from build123d import *

# Parameters (mm, degrees)
BOSS_EXTRUDE1_DEPTH = 5
CUT_EXTRUDE3_DEPTH  = 2


with BuildPart() as part:
    # Sketch1 → Boss-Extrude1 (new body)
    with BuildSketch(Plane(origin=(0, 0, 0), x_dir=(0, 0, -1), z_dir=(1, 0, 0))):
        with BuildLine():
            Line((-25, 10), (25, 10))
            Line((25, 10), (25, -10))
            Line((25, -10), (-25, -10))
            ThreePointArc((-25, -10), (-35, 0), (-25, 10))
        make_face()
    extrude(amount=BOSS_EXTRUDE1_DEPTH)

    # Sketch2 → Cut-Extrude3 (cut)
    with BuildSketch(Plane(origin=(5, 0, 0), x_dir=(0, 0, -1), z_dir=(1, 0, 0))):
        with BuildLine():
            ThreePointArc((-21, 0), (-22.171572875, 2.828427125), (-25, 4))
            Line((-25, 4), (-25, -4))
            ThreePointArc((-25, -4), (-22.171572875, -2.828427125), (-21, 0))
        make_face()
        with BuildLine():
            Line((-25, -4), (-25, 4))
            ThreePointArc((-25, 4), (-29, 0), (-25, -4))
        make_face()
    extrude(amount=-CUT_EXTRUDE3_DEPTH, mode=Mode.SUBTRACT)


solid = part.part
CAD build for the part. Positions are in the model's coordinates, mm. Coordinates: 2 decimals unless noted, no trailing zeros. Write each loop counter-clockwise with the first axis right and the second up, starting at its lowest first coordinate (ties: lowest second). Pieces come first, ordered by that corner, then holes. Notation, with made-up numbers: M 47.25,-38 L 99.25,-38 A22 ccw 99.25,-18 Z; hole C 56.25,-27.75 d10. An arc over 180 degrees is marked long. Return JSON: item names as keys, results as strings.
Item 1: Slice it at B-B, the plane y = 2.5. Write the cut outline in (x, z).
Findings below:
{"outline": "M 0,-25 L 5,-25 L 5,21.88 L 3,21.88 L 3,28.12 L 5,28.12 L 5,34.68 L 0,34.68 Z"}
Item 2: Drop a flat-ended pin along its axis: pin 1 Ø4 at (y, z) = (-1, 25.5) entering from +X. Give the stop position or say it passes through.
Findings below:
{"pin 1": "stops at x = 3"}
Item 3: Slice it at D-D, the plane x = 0.6. Write the cut outline in (y, z).
Findings below:
{"outline": "M -10,-25 L 10,-25 L 10,25 A10 ccw -10,25 Z"}
Item 4: Two-plate mould, pull along Z, no slides. Class faces 1 (the flat face through (2, 0, -25)), 2 (the cylindrical face through (2, 0, 35)), 3 (the flat face through (5, 0, 5)), 4 (the flat face through (3, 0, 25)): +Z half, -Z half, draft (parallel to the pull), parting line (faces both ways), or undercut.
Findings below:
{"face 1": "-Z half", "face 2": "+Z half", "face 3": "draft", "face 4": "undercut"}
Item 5: Slice it at A-A, the plane x = 4.4. Write the cut outline in (y, z).
Findings below:
{"outline": "M -10,-25 L 10,-25 L 10,25 A10 ccw -10,25 Z; hole C 0,25 d8"}
Item 6: Slice it at C-C, the plane z = 31. Write the cut outline in (x, y), and give its area (3 significant figures).
Findings below:
{"outline": "M 0,-8 L 5,-8 L 5,8 L 0,8 Z", "area": "80.0 mm2"}
Item 7: Probe line 1 (Z direction, x = 4.4, y = -1.5); line 2 (Z direction, x = 4.5, y = 3.5); line 3 (Z direction, x = 2.4, y = -4.75). List the from-to ranges inside material, lowest first. Write a range as from..to.
Findings below:
{"line 1": "z = -25..21.29, 28.71..34.89", "line 2": "z = -25..23.06, 26.94..34.37", "line 3": "z = -25..33.8"}
